Verification items for this drawing (mm, ordinates from the low corner). A direction names the side the tool comes from. Round coordinates to 2 decimals unless told otherwise and drop trailing zeros. Loops run counter-clockwise (first coordinate to the right, second up) from the corner with the lowest first, then second, coordinate; pieces in that order, holes last. Notation, with made-up numbers: (41, -28) - (99, -28) arc R36 ccw to (99, 9) - close; hole circle Ø1 at (31.25, 40). An arc over 180 degrees is marked (long way). Put each result on its own line as item: value. Start each with the question number.
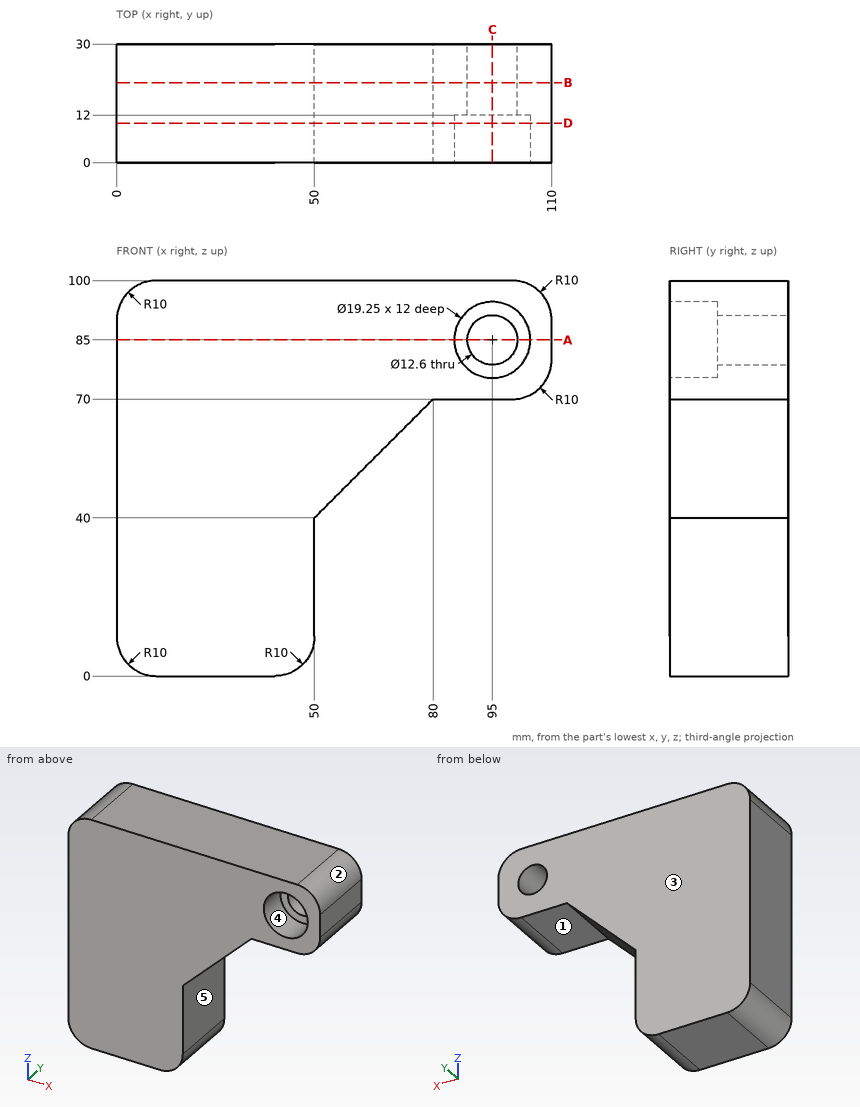
Q1. Draft check along X on the marked faces 3, 4 and 5. Enter one of: +X half, -X half, draft (parallel to the pull), parting line (faces both ways), or undercut.
Q2. Cross-section at D-D on y = 10. Enter the section's corners in (x, z) (3 decimals).
Q3. Cross-section at A-A on z = 85. Enter the section's corners in (x, y) (3 decimals), and give its area (3 significant figures).
Q4. Depth check by flat-ended pin: pin 1 Ø12 at (x, y) = (48, 15.5) entering from -Z; pin 2 Ø9 at (y, z) = (12, 24.5) entering from +X; pin 3 Ø17.5 at (x, z) = (95, 85) entering from -Y; pin 4 Ø7.5 at (x, z) = (95, 85) entering from +Y. Enter the tip coordinate at first touch or a pass-through.
Q5. Set-up check for the marked faces 1 and 2: record each of +Z, -Z, +X, -X, +Y, -Y from which the full face is reachable in a straight line by a thin tool's end or side.
Q6. Material ranges on line 1 (Z direction, x = 95, y = 24.75); line 2 (Z direction, x = 81, y = 26.25); line 3 (Z direction, x = 95, y = 6.5) (3 decimals), recorded low to high. Write a range as from..to.
Q7. Cross-section at C-C on x = 95. Enter the section's corners in (y, z) (3 decimals).
Q8. Cross-section at B-B on y = 20.25. Enter the section's corners in (x, z).
Answer list:
1. face 3: draft
1. face 4: undercut
1. face 5: +X half
2. outline: (0, 10) arc R10 ccw to (10, 0) - (40, 0) arc R10 ccw to (50, 10) - (50, 40) - (80, 70) - (100, 70) arc R10 ccw to (110, 80) - (110, 90) arc R10 ccw to (100, 100) - (10, 100) arc R10 ccw to (0, 90) - close; hole circle Ø19.25 at (95, 85)
3. outline: (0, 0) - (85.375, 0) - (85.375, 12) - (88.7, 12) - (88.7, 30) - (0, 30) - close; (101.3, 12) - (104.625, 12) - (104.625, 0) - (110, 0) - (110, 30) - (101.3, 30) - close
3. area: 2,840 mm2
4. pin 1: stops at z = 0.2
4. pin 2: stops at x = 50
4. pin 3: stops at y = 12
4. pin 4: passes through
5. face 1: -Z, +X, +Y, -Y
5. face 2: +Z, +X, +Y, -Y
6. line 1: z = 70..78.7, 91.3..100
6. line 2: z = 70..100
6. line 3: z = 70..75.375, 94.625..100
7. outline: (0, 70) - (30, 70) - (30, 78.7) - (12, 78.7) - (12, 75.375) - (0, 75.375) - close; (0, 94.625) - (12, 94.625) - (12, 91.3) - (30, 91.3) - (30, 100) - (0, 100) - close
8. outline: (0, 10) arc R10 ccw to (10, 0) - (40, 0) arc R10 ccw to (50, 10) - (50, 40) - (80, 70) - (100, 70) arc R10 ccw to (110, 80) - (110, 90) arc R10 ccw to (100, 100) - (10, 100) arc R10 ccw to (0, 90) - close; hole circle Ø12.6 at (95, 85)
